Geometry check sheet. Reference: the model listing, model coordinates, mm. Round coordinates to 2 decimals unless told otherwise and drop trailing zeros. Write each loop counter-clockwise with the first axis right and the second up, starting at its lowest first coordinate (ties: lowest second). Pieces come first, ordered by that corner, then holes.
Item 1: Scan lines: probe 1 along X at (y, z) = (1, -0.75) (3 decimals); probe 2 along Z at (x, y) = (70.5, 1.5); probe 3 along Z at (x, y) = (59, 0.75). Record each from-to range of solid material in increasing order.
Item 2: Depth check by flat-ended pin: P1, Ø1.7, axis at y = 2, z = 0, coming from the +X side (3 decimals); P2, Ø1.5, axis at x = 74, y = 2, coming from the +Z side; P3, Ø1.5, axis at y = -2, z = -1, coming from the -X side. Enter the tip coordinate at first touch or a pass-through.
Item 3: Cross-section at A-A (x = 0). Enter the section's corners in (y, z), then the cut area to 3 significant figures.
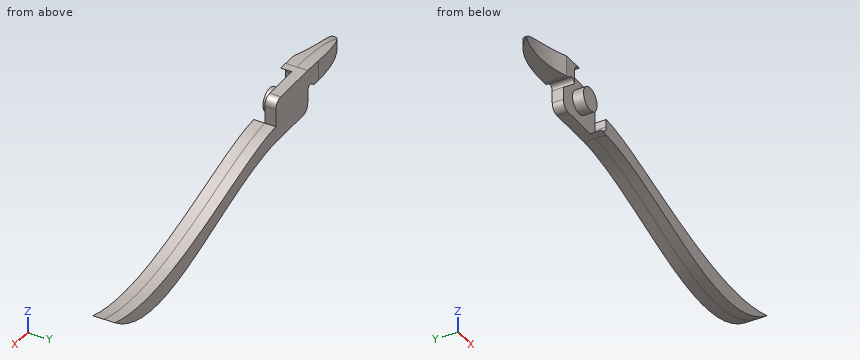
from build123d import *

# Parameters (mm, degrees)
SKETCH1_R                = 3.4925
BOSS_EXTRUDE3_DEPTH      = 3.302
BOSS_EXTRUDE4_DEPTH      = 3.302
BOSS_EXTRUDE5_DEPTH      = 3.302
CUT_EXTRUDE1_REACH       = 8.35
SKETCH1_11_R             = 3.4925
BOSS_EXTRUDE6_DEPTH      = 3.302
BOSS_EXTRUDE6_DEPTH_BACK = 3.302


with BuildPart() as part:
    # Sketch1 → Boss-Extrude3 (new body)
    with BuildSketch(Plane(origin=(0, 0, 0), x_dir=(1, 0, 0), z_dir=(0, 1, 0))):
        with BuildLine():
            ThreePointArc((-10.47160211, -0.846666667), (-11.327855674, -0.22130784), (-12.364806331, 0))
            Line((-12.364806331, 0), (-33.02, 0))
            add(Edge.make_bspline(
                [(-33.02, 0), (-27.473096433, -6.223159861), (-8.255, -6.35)],
                knots=[0, 0, 0, 1, 1, 1], degree=2))
            Line((-8.255, -6.35), (-8.255, -3.81))
            Line((-8.255, -3.81), (-8.255, 0))
            ThreePointArc((-8.255, 0), (-9.071835946, -1.186398896), (-10.47160211, -0.846666667))
        make_face()
        with BuildLine():
            ThreePointArc((5.715, 6.35), (7.511051224, 5.606051224), (8.255, 3.81))
            Line((8.255, 3.81), (8.255, -3.81))
            ThreePointArc((8.255, -3.81), (7.511051224, -5.606051224), (5.715, -6.35))
            Line((5.715, -6.35), (-5.715, -6.35))
            ThreePointArc((-5.715, -6.35), (-7.511051224, -5.606051224), (-8.255, -3.81))
            Line((-8.255, -3.81), (-8.255, 3.81))
            ThreePointArc((-8.255, 3.81), (-7.511051224, 5.606051224), (-5.715, 6.35))
            Line((-5.715, 6.35), (5.715, 6.35))
        make_face()
        with Locations(Location((0, 0, 0), (0, 0, 270))):  # turned: the seam where the file's is
            Circle(SKETCH1_R, mode=Mode.SUBTRACT)
        with BuildLine():
            ThreePointArc((-8.255, -3.81), (-7.511051224, -5.606051224), (-5.715, -6.35))
            Line((-5.715, -6.35), (-8.255, -6.35))
            Line((-8.255, -6.35), (-8.255, -3.81))
        make_face()
        with BuildLine():
            Line((8.255, 3.527942587), (8.255, 1.524))
            add(Edge.make_bspline(
                [(8.255, 1.524), (26.922144182, 2.150849617), (62.646246262, 22.822886738), (91.44, 13.97)],
                knots=[0, 0, 0, 0, 1, 1, 1, 1], degree=3))
            add(Edge.make_bspline(
                [(91.44, 13.97), (66.350363848, 33.352051218), (36.841337127, 7.764653999), (8.255, 6.35)],
                knots=[0, 0, 0, 0, 1, 1, 1, 1], degree=3))
            Line((8.255, 6.35), (8.255, 3.81))
            Line((8.255, 3.81), (8.255, 3.527942587))
        make_face()
        with BuildLine():
            Line((8.255, 6.35), (5.715, 6.35))
            ThreePointArc((5.715, 6.35), (7.511051224, 5.606051224), (8.255, 3.81))
            Line((8.255, 3.81), (8.255, 6.35))
        make_face()
    extrude(amount=BOSS_EXTRUDE3_DEPTH)

    # Sketch1_8 → Boss-Extrude4 (add)
    with BuildSketch(Plane(origin=(0, 0, 0), x_dir=(1, 0, 0), z_dir=(0, 1, 0))):
        with BuildLine():
            Line((8.255, 3.527942587), (8.255, 1.524))
            add(Edge.make_bspline(
                [(8.255, 1.524), (26.922144182, 2.150849617), (62.646246262, 22.822886738), (91.44, 13.97)],
                knots=[0, 0, 0, 0, 1, 1, 1, 1], degree=3))
            add(Edge.make_bspline(
                [(91.44, 13.97), (66.350363848, 33.352051218), (36.841337127, 7.764653999), (8.255, 6.35)],
                knots=[0, 0, 0, 0, 1, 1, 1, 1], degree=3))
            Line((8.255, 6.35), (8.255, 3.81))
            Line((8.255, 3.81), (8.255, 3.527942587))
        make_face()
        with BuildLine():
            Line((8.255, 6.35), (5.715, 6.35))
            ThreePointArc((5.715, 6.35), (7.511051224, 5.606051224), (8.255, 3.81))
            Line((8.255, 3.81), (8.255, 6.35))
        make_face()
    extrude(amount=-BOSS_EXTRUDE4_DEPTH)

    # Sketch1_9 → Boss-Extrude5 (add)
    with BuildSketch(Plane(origin=(0, 0, 0), x_dir=(1, 0, 0), z_dir=(0, 1, 0))):
        with BuildLine():
            ThreePointArc((-10.47160211, -0.846666667), (-11.327855674, -0.22130784), (-12.364806331, 0))
            Line((-12.364806331, 0), (-33.02, 0))
            add(Edge.make_bspline(
                [(-33.02, 0), (-27.473096433, -6.223159861), (-8.255, -6.35)],
                knots=[0, 0, 0, 1, 1, 1], degree=2))
            Line((-8.255, -6.35), (-8.255, -3.81))
            Line((-8.255, -3.81), (-8.255, 0))
            ThreePointArc((-8.255, 0), (-9.071835946, -1.186398896), (-10.47160211, -0.846666667))
        make_face()
        with BuildLine():
            ThreePointArc((-8.255, -3.81), (-7.511051224, -5.606051224), (-5.715, -6.35))
            Line((-5.715, -6.35), (-8.255, -6.35))
            Line((-8.255, -6.35), (-8.255, -3.81))
        make_face()
    extrude(amount=-BOSS_EXTRUDE5_DEPTH)

    # Sketch2 → Cut-Extrude1 (cut, up to next)
    with BuildSketch(Plane.XY, mode=Mode.PRIVATE) as cut_extrude1_sk1:
        with BuildLine():
            Line((-33.02, 3.302), (-33.02, -3.053994927))
            add(Edge.make_bspline(
                [(-33.02, -3.053994927), (-28.519594092, 1.640722514), (-22.101826858, 3.211473856), (-13.921878912, 3.302)],
                knots=[0, 0, 0, 0, 0.941080878, 0.941080878, 0.941080878, 0.941080878], degree=3))
            Line((-13.921878912, 3.302), (-33.02, 3.302))
        make_face()
    cut_extrude1_tool1 = extrude(cut_extrude1_sk1.sketch, amount=CUT_EXTRUDE1_REACH, mode=Mode.PRIVATE) & part.part
    add(cut_extrude1_tool1.solids().sort_by_distance((-28.707051, 1.545014, 0))[0], mode=Mode.SUBTRACT)
    # Sketch2 → Cut-Extrude1 (cut, up to next)
    with BuildSketch(Plane.XY, mode=Mode.PRIVATE) as cut_extrude1_sk2:
        with BuildLine():
            Line((-12.364806331, -3.302), (-33.02, -3.302))
            add(Edge.make_bspline(
                [(-12.364806331, -3.302), (-18.804874471, -1.031483357), (-26.812471442, -0.753963495), (-33.02, -3.302)],
                knots=[0, 0, 0, 0, 1, 1, 1, 1], degree=3))
        make_face()
    cut_extrude1_tool2 = extrude(cut_extrude1_sk2.sketch, amount=CUT_EXTRUDE1_REACH, mode=Mode.PRIVATE) & part.part
    add(cut_extrude1_tool2.solids().sort_by_distance((-22.84596, -2.573969, 0))[0], mode=Mode.SUBTRACT)

    # Sketch1_11 → Boss-Extrude6 (add, two sides)
    with BuildSketch(Plane(origin=(0, 0, 0), x_dir=(1, 0, 0), z_dir=(0, 1, 0))) as boss_extrude6_sk:
        with Locations(Location((0, 0, 0), (0, 0, 270))):  # turned: the seam where the file's is
            Circle(SKETCH1_11_R)
    extrude(amount=BOSS_EXTRUDE6_DEPTH)
    extrude(boss_extrude6_sk.sketch, amount=-BOSS_EXTRUDE6_DEPTH_BACK)


solid = part.part
Resolved:
1. probe 1: x = -8.255 to 8.255
1. probe 2: z = -21.19 to -15.98
1. probe 3: z = -19.96 to -14.41
2. P1: stops at x = 8.255
2. P2: stops at z = -16.13
2. P3: stops at x = -3.48
3. outline: (-3.3, -3.49) - (0, -3.49) - (0, -6.35) - (3.3, -6.35) - (3.3, 6.35) - (0, 6.35) - (0, 3.49) - (-3.3, 3.49) - close
3. area: 65.0 mm2
